Input: part model. Units: mm. Frame: model coordinates. Give positions to 0.01 mm unless a question says otherwise; leave off trailing zeros. Loops run counter-clockwise (first coordinate to the right, second up) from the corner with the lowest first, then second, coordinate; pieces in that order, holes last. Notation, with made-up numbers: (71.25, 33) - (102.25, 33) arc R23 cw to (102.25, 63) - close; hole circle Ø10 at (2, 33). An arc over 180 degrees is marked (long way). Answer as a JSON object with one key per item and string values. Group by question number.
(1) Section query B-B (z = 20.5). Return loops of the section in (x, y), plus the area to 3 significant figures.
(2) Pin query (flat end, axial travel): P1, Ø0.8, axis at x = 24, y = 1, coming from the +Z side. Return the tip coordinate at first contact, or that it passes through.
(3) Section query A-A (y = 1.3). Return loops of the section in (x, z), plus the area to 3 significant figures.
(4) Material intervals for L1, parallel to Z at x = 45, y = 1.45; L2, parallel to X at y = 1, z = 13.5, sorted ascending.
(5) Section query C-C (x = 15). Return loops of the section in (y, z).
Autodesk Inventor part; units mm, degrees
ref_plane "YZ Plane" through (0, 0, 0) normal (1, 0, 0) x (0, 1, 0)
ref_plane "XZ Plane" through (0, 0, 0) normal (0, 1, 0) x (-1, 0, 0)
ref_plane "XY Plane" through (0, 0, 0) normal (0, 0, 1) x (1, 0, 0)
sketch "Sketch1" plane through (0, 0, 0) normal (0, 1, 0) x (-1, 0, 0)
  line L0 (-50, 10.5) -> (3, 10.5)
  line L1 (50, -2.7166) -> (50, -10.5)
  line L2 (50, -10.5) -> (-50, -10.5)
  line L3 (-50, -10.5) -> (-50, 10.5)
  line L4 (50, -2.7166) -> (50, 27.5)
  line L5 (50, 27.5) -> (3, 27.5)
  line L6 (3, 27.5) -> (3, 10.5)
  point P0 (0, 0)
  dimension "d0" = 47
  dimension "d1" = 17
  dimension "d2" = 100
  dimension "d3" = 21
  dimension "d4" = 10.5
  dimension "d5" = 50
extrude "Extrusion1" add sketch "Sketch1" along normal blind 1.6
properties part number "pcb"
Recorded:
{
 "1": {"outline": "(-50, 0) - (-3, 0) - (-3, 1.6) - (-50, 1.6) - close", "area": "75.2 mm^2"},
 "2": {"P1": "stops at z = 10.5"},
 "3": {"outline": "(-50, -10.5) - (50, -10.5) - (50, 10.5) - (-3, 10.5) - (-3, 27.5) - (-50, 27.5) - close", "area": "2,900 mm^2"},
 "4": {"L1": "z = -10.5 to 10.5", "L2": "x = -50 to -3"},
 "5": {"outline": "(0, -10.5) - (1.6, -10.5) - (1.6, 10.5) - (0, 10.5) - close"}
}
